```python
from build123d import *

# Parameters (mm, degrees)
F1_DEPTH = 127
F2_R     = 25.4
F3_DEPTH = 152.4


with BuildPart() as f1:
    # F0 (on Right) → F1 (new body)
    with BuildSketch(Plane.YZ):
        Polygon((63.745255, 56.260998), (-88.654745, 56.260998), (-88.654745, -70.739002), (-63.254745, -70.739002), (-63.254745, 30.860998), (38.345255, 30.860998), (38.345255, -70.739002), (63.745255, -70.739002), align=None)
    extrude(amount=F1_DEPTH)

    # F2 (on face) → F3 (join)
    with BuildSketch(Plane.XZ.offset(88.654745)):
        with Locations((64.692467, -26.329797)):
            Circle(F2_R)
    extrude(amount=-F3_DEPTH)


solid = f1.part
```
Geometry check sheet. Reference: the model listing, model coordinates, mm. A direction names the side the tool comes from. Round coordinates to 2 decimals unless told otherwise and drop trailing zeros. Write each loop counter-clockwise with the first axis right and the second up, starting at its lowest first coordinate (ties: lowest second). Pieces come first, ordered by that corner, then holes. Notation, with made-up numbers: (17, 58) -> (48, 58) arc R9 cw to (48, 65) -> close; hole circle Ø2 at (-23, 77.25). An arc over 180 degrees is marked (long way). Put each result on its own line as item: value.
1) Cross-section at A-A, the plane z = 21. Enter the section's corners in (x, y).
Recorded:
outline: (0, -88.65) -> (127, -88.65) -> (127, -63.25) -> (0, -63.25) -> close; (0, 38.35) -> (127, 38.35) -> (127, 63.75) -> (0, 63.75) -> close
2) Cross-section at B-B, the plane x = 80. Enter the section's corners in (y, z), plus the area to 3 significant figures.
Recorded:
outline: (-88.65, -70.74) -> (-63.25, -70.74) -> (-63.25, -46.6) -> (38.35, -46.6) -> (38.35, -70.74) -> (63.75, -70.74) -> (63.75, 56.26) -> (-88.65, 56.26) -> close; hole (-63.25, -6.06) -> (38.35, -6.06) -> (38.35, 30.86) -> (-63.25, 30.86) -> close
area: 13,200 mm2
3) Thickness scan on probe 1 along Y at (x, z) = (59, 12.5); probe 2 along Z at (x, y) = (24.5, 9.5); probe 3 along Z at (x, y) = (58, -5). Record the ranges inside material, lowest first. Write a range as from..to.
Recorded:
probe 1: y = -88.65..-63.25, 38.35..63.75
probe 2: z = 30.86..56.26
probe 3: z = -50.83..-1.83, 30.86..56.26
4) Access from +Z, -Z, +X, -X, +Y, -Y to the whole of each face (thin tool, end or side, straight path). Record for faces 1 (the face through (63, -63.255, 2)), 2 (the face through (63, -76, -70.739)).
Recorded:
face 1: none
face 2: -Z, +X, -X, +Y, -Y
5) Release check for a two-part mould opening along Y. For faces 3 (the face through (88.92, -13.17, -18.7)), 4 (the face through (63, -13, 30.861)), 5 (the face through (63, 51, -70.739)), 6 (the face through (63, -88.655, -6)) record: pulls with the +Y half, pulls with the -Y half, needs draft (parallel to the pull), parting line crosses it, or undercut.
Recorded:
face 3: undercut
face 4: undercut
face 5: needs draft
face 6: pulls with the -Y half
6) Cross-section at D-D, the plane x = 32. Enter the section's corners in (y, z).
Recorded:
outline: (-88.65, -70.74) -> (-63.25, -70.74) -> (-63.25, 30.86) -> (38.35, 30.86) -> (38.35, -70.74) -> (63.75, -70.74) -> (63.75, 56.26) -> (-88.65, 56.26) -> close
7) Cross-section at C-C, the plane y = -12. Enter the section's corners in (x, z), plus the area to 3 significant figures.
Recorded:
outline: (0, 30.86) -> (127, 30.86) -> (127, 56.26) -> (0, 56.26) -> close; circle Ø50.8 at (64.69, -26.33)
area: 5,250 mm2
